Part model, mm, in its own coordinate system. A direction names the side the tool comes from. Round coordinates to 2 decimals unless told otherwise and drop trailing zeros. Loops run counter-clockwise (first coordinate to the right, second up) from the corner with the lowest first, then second, coordinate; pieces in that order, holes last. Notation, with made-up numbers: (-7.5, -21) - (-3.5, -21) arc R33 ccw to (-3.5, 8) - close; hole circle Ø7 at (52.5, 56.25). An arc over 180 degrees is marked (long way). Put each result on its own line as item: value.
from build123d import *

# Parameters (mm, degrees)
F0_W     = 50
F0_H     = 50
F1_DEPTH = 25
F2_R     = 5
F3_DEPTH = 10


with BuildPart() as f1:
    # F0 (on Front) → F1 (new body)
    with BuildSketch(Plane.XZ):
        Rectangle(F0_W, F0_H)
    extrude(amount=-F1_DEPTH)

    # F2 (on face) → F3 (join)
    with BuildSketch(Plane.XZ):
        Circle(F2_R)
    extrude(amount=F3_DEPTH)


solid = f1.part
1. Probe line 1 along Y through (x, z) = (22.5, -8); line 2 along Z through (x, y) = (-0.5, -4). List the from-to ranges inside material, lowest first. Write a range as [from, to].
A:
line 1: y = [0, 25]
line 2: z = [-4.97, 4.97]
2. Pin check, flat tips, straight feed: P1, Ø25, axis at x = 9.5, z = -12, coming from the -Y side; P2, Ø5, axis at x = 11.5, z = 5, coming from the -Y side. Stop position of each tip, or through.
A:
P1: stops at y = -10
P2: stops at y = 0
3. Band-saw the part on C-C (y = -5). List the corners of the cut face in (x, z).
A:
outline: circle Ø10 at (0, 0)
4. Tool access for faces 1 (the cylindrical face through (-1.08, -4.93, -4.88)), 2 (the flat face through (0, -10, 0)): list every direction of +Z, -Z, +X, -X, +Y, -Y with a clear straight run to the whole face (end or side of a thin tool).
A:
face 1: -Y
face 2: +Z, -Z, +X, -X, -Y
5. Band-saw the part on D-D (z = -15.5). List the corners of the cut face in (x, y), plus the area to 3 significant figures.
A:
outline: (-25, 0) - (25, 0) - (25, 25) - (-25, 25) - close
area: 1,250 mm²
6. Band-saw the part on B-B (z = 0). List the corners of the cut face in (x, y).
A:
outline: (-25, 0) - (-5, 0) - (-5, -10) - (5, -10) - (5, 0) - (25, 0) - (25, 25) - (-25, 25) - close
7. Band-saw the part on A-A (x = 0). List the corners of the cut face in (y, z).
A:
outline: (-10, -5) - (0, -5) - (0, -25) - (25, -25) - (25, 25) - (0, 25) - (0, 5) - (-10, 5) - close
